Can you work these out from the model? Positions are in its coordinate system, mm. Face numbers are marked on the shaded views. A direction names the side the tool comes from. Coordinates: 2 decimals unless noted, no trailing zeros. Write each loop counter-clockwise with the first axis right and the second up, starting at its lowest first coordinate (ties: lowest second). Pieces come first, ordered by that corner, then holes. Notation, with made-up numbers: (77.25, 4) -> (104.25, 4) arc R10 cw to (104.25, 10) -> close; hole circle Ø7 at (23.25, -38). An arc over 180 degrees is marked (long way). Use one line per item in the form item = value.
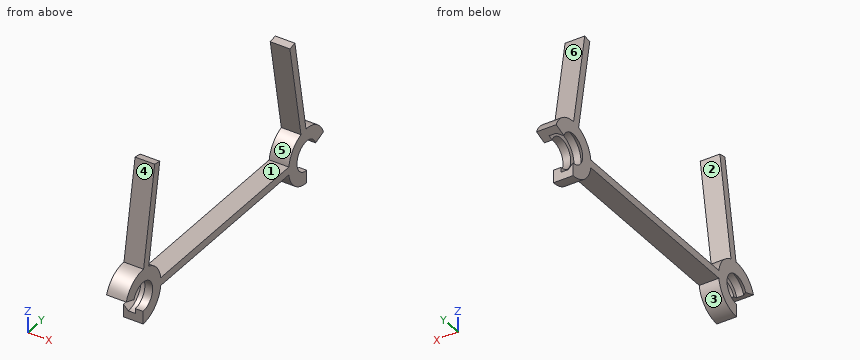
Autodesk Inventor part; units mm, degrees
ref_plane "Work Plane1" through (-2, 20, -2.8) normal (0, -1, 0) x (1, 0, 0)
ref_plane "YZ Plane" through (0, 0, 0) normal (1, 0, 0) x (0, 1, 0)
ref_plane "XZ Plane" through (0, 0, 0) normal (0, 1, 0) x (-1, 0, 0)
sketch "Sketch1" plane through (0, 0, 0) normal (0, 1, 0) x (-1, 0, 0)
  line L0 (2, -1.5) -> (1.5, -2)
  line L1 (1.5, -2) -> (0.79, -2)
  line L2 (0.79, -2) -> (0.79, -1.5)
  line L3 (0.79, -1.5) -> (0, -1.5)
  line L4 (0, -1.5) -> (0, -2.8)
  line L5 (0, -2.8) -> (2, -2.8)
  line L6 (2, -2.8) -> (2, -1.5)
  line L7 (0, 0) -> (1.5115, 0)
  line L8 (2, -12.5) -> (2, -13.8)
  line L9 (2, -13.8) -> (0, -13.8)
  line L10 (0, -13.8) -> (0, -12.5)
  line L11 (0, -12.5) -> (0.5, -13)
  line L12 (0.5, -13) -> (1.5, -13)
  line L13 (1.5, -13) -> (2, -12.5)
  line L14 (0, -10) -> (1, -10)
  point P0 (1, -13)
  dimension "d0" = 0.5
  dimension "d1" = 45
  dimension "d2" = 0.8
  dimension "d3" = 0.71
  dimension "d5" = 2
  dimension "d6" = 1
  dimension "d7" = 0.8
  dimension "d8" = 0.5
  dimension "d9" = 10
  dimension "d10" = 3
revolve "Revolution1" add sketch "Sketch1" angle 250 about axis through (0, 0, 0) along (1, 0, 0) contours L6 L5 L4 L3 L2 L1 L0
sketch "Sketch3" plane through (-2, 0, -2.8) normal (-1, 0, 0) x (0, 0, 1)
  arc A0 (3.7577, -2.6311) -> (0, 0) centre (2.8, 0) ccw
  line L0 (2.4, 2.7713) -> (2.4, 12.7713)
  line L1 (2.4, 12.7713) -> (3.2, 12.7713)
  line L2 (3.2, 12.7713) -> (3.2, 2.7713)
  line L3 (5.4597, 0.8752) -> (15.3078, 2.6116)
  line L4 (15.3078, 2.6116) -> (15.4467, 1.8238)
  line L5 (15.4467, 1.8238) -> (5.5986, 0.0873)
  point P0 (2.8, 0)
  dimension "d31" = 0.8
  dimension "d32" = 10
  dimension "d33" = 80
  dimension "d14" = 0.81
  dimension "d16" = 2
  dimension "d18" = 2
  dimension "d19" = 0.81
  dimension "d20" = 70
  dimension "d27" = 1.356
  dimension "d28" = 0.8
extrude "Extrusion4" add sketch "Sketch3" against normal up to surface (2 mm away)
mirror "Mirror3" about plane through (-2, 12.7713, -0.4) normal (0, 1, 0) of "Extrusion4", "Revolution1"
properties part number "lens mounts"
Q1. Suppose I cut it at A-A (z = 0). Write out the boundary of the cut face in (x, y).
Return value:
outline = (-2, 1.5) -> (-1.5, 2) -> (-0.79, 2) -> (-0.79, 1.5) -> (0, 1.5) -> (0, 24.04) -> (-0.79, 24.04) -> (-0.79, 23.54) -> (-1.5, 23.54) -> (-2, 24.04) -> close
Q2. Suppose I cut it at B-B (z = 11.25). Write out the boundary of the cut face in (x, y), then the cut area to 3 significant figures.
Return value:
outline = (-2, 1.58) -> (0, 1.58) -> (0, 2.39) -> (-2, 2.39) -> close; (-2, 23.15) -> (0, 23.15) -> (0, 23.97) -> (-2, 23.97) -> close
area = 3.25 mm2
Q3. Will these pins go through, and if not, where does the flat tip stop? pin 1 (0.6 mm diameter, centred on x = -1, y = 17.5, fed in from +Z); pin 2 (0.6 mm diameter, centred on x = -0.5, y = 16, fed in from -Z); pin 3 (0.6 mm diameter, centred on x = -0.5, z = -2, fed in from -Y).
Return value:
pin_1 = 0.4
pin_2 = -0.4
pin_3 = 0
Q4. If I drill on line 1 (Y direction, x = -1, z = 0); line 2 (Y direction, x = -0.2, z = 0); line 3 (Y direction, x = -1.15, z = 9.5), over which ranges is the centre line in solid material (lowest first)? Write a range as from..to.
Return value:
line_1 = 2..23.54
line_2 = 1.5..24.04
line_3 = 1.27..2.08, 23.46..24.27
Q5. For the marked faces 1, 2 and 3, which set-ups out of +Z, -Z, +X, -X, +Y, -Y let a thin tool reach every point of the face, with its end or its side?
Return value:
face_1 = +Z, +X, -X
face_2 = +X, -X
face_3 = -Z, +X, -X
Q6. Suppose I cut it at C-C (x = -0.4). Write out the boundary of the cut face in (y, z).
Return value:
outline = (-2.63, 0.96) -> (-1.41, 0.51) arc R1.5 cw (long way) to (0, -1.5) -> (0, -2.8) arc R2.8 ccw to (2.77, -0.4) -> (22.77, -0.4) arc R2.8 ccw to (25.54, -2.8) -> (25.54, -1.5) arc R1.5 cw (long way) to (26.95, 0.51) -> (28.17, 0.96) arc R2.8 ccw to (25.46, 2.8) -> (23.72, 12.65) -> (22.93, 12.51) -> (24.67, 2.66) arc R2.8 ccw to (22.77, 0.4) -> (2.77, 0.4) arc R2.8 ccw to (0.88, 2.66) -> (2.61, 12.51) -> (1.82, 12.65) -> (0.09, 2.8) arc R2.8 ccw to start
Q7. Suppose I cut it at D-D (y = 7.5). Write out the boundary of the cut face in (x, z), then the cut area to 3 significant figures.
Return value:
outline = (-2, -0.4) -> (0, -0.4) -> (0, 0.4) -> (-2, 0.4) -> close
area = 1.60 mm2
Q8. Thinking about a two-plate mould opening in Y: for the marked faces 4, 5 and 6, which applies, released by +Y, released by -Y, zero draft, split by the parting line, or undercut?
Return value:
face_4 = released by -Y
face_5 = undercut
face_6 = released by +Y
